Source: CAD feature listing. Evaluate the final solid. Frame: model axes, mm. A direction names the side the tool comes from. Give positions to 0.01 mm unless a question says otherwise; leave off trailing zeros. Write each loop counter-clockwise with the first axis right and the second up, starting at its lowest first coordinate (ties: lowest second). Pieces come first, ordered by that corner, then holes. Notation, with made-up numbers: (-26.75, 72.5) -> (-20.75, 72.5) arc R5 cw to (-20.75, 76.5) -> close; hole circle Ø7 at (-4.5, 49). An arc over 180 degrees is marked (long way). Use one line per item in the form item = value. Start each with the question number.
(1) Set-up query: faces 1 (the face through (35, 0, 23)), 2 (the face through (23.65, -49.45, -25.8)), 3 (the face through (15.02, 271.03, 47.69)), 4 (the face through (35, 0, -25)). Return all of +Z, -Z, +X, -X, +Y, -Y with unobstructed straight access to the full face (end or side cutting, diameter ignored); none if empty.
(2) Cut plane B-B, the plane z = -8. Output: boundary loops of the cut face in (x, y).
(3) Cut plane C-C, the plane y = 370. Output: boundary loops of the cut face in (x, z), and give its area (3 significant figures).
(4) Material intervals for line 1 along X through (y, z) = (0, -1); line 2 along X through (y, z) = (1.5, 18.5); line 3 along Y through (x, z) = (0, -15), sorted ascending. Write a range as from..to.
(5) Cut plane D-D, the plane y = -26.5. Output: boundary loops of the cut face in (x, z), and give its area (3 significant figures).
(6) First-contact query: P1, Ø2, axis at x = 7.5, y = 228.5, coming from the +Z side; P2, Ø6, axis at y = 285, z = -0.5, coming from the +X side; P3, Ø8, axis at x = -29, y = 278, coming from the +Z side. Flat tips, straight axial feed; report the tip coordinate or a pass-through.
(7) Cut plane A-A, the plane x = 15. Output: boundary loops of the cut face in (y, z), and give its area (3 significant figures).
from build123d import *

# Parameters (mm, degrees)
BOSS_EXTRUDE1_DEPTH      = 132
BOSS_EXTRUDE1_DEPTH_BACK = 80
SKETCH1_R                = 35
BOSS_EXTRUDE2_DEPTH      = 35
BOSS_EXTRUDE2_DEPTH_BACK = 35
SKETCH2_R                = 35
SKETCH3_R                = 52.5
BOSS_EXTRUDE3_DEPTH      = 20
SKETCH4_R                = 50
BOSS_EXTRUDE4_DEPTH      = 282
CUT_EXTRUDE1_DEPTH       = 427.390079622
CUT_EXTRUDE1_DEPTH_BACK  = 427.390079622
SKETCH5_R                = 20


with BuildPart() as part:
    # Sketch1 → Boss-Extrude1 (new, two sides: drawn at the far end of the back side and taken through both)
    with BuildSketch(Plane(origin=(0, 0, 0), x_dir=(1, 0, 0), z_dir=(0, 1, 0)).offset(-BOSS_EXTRUDE1_DEPTH_BACK)):
        with Locations(Location((0, 0, 0), (0, 0, 270))):
            Circle(SKETCH1_R)
    extrude(amount=BOSS_EXTRUDE1_DEPTH + BOSS_EXTRUDE1_DEPTH_BACK)

    # Sketch2 → Boss-Extrude2 (add, two sides: drawn at the far end of the back side and taken through both)
    with BuildSketch(Plane.XY.offset(-BOSS_EXTRUDE2_DEPTH_BACK)):
        Circle(SKETCH2_R)
    extrude(amount=BOSS_EXTRUDE2_DEPTH + BOSS_EXTRUDE2_DEPTH_BACK)

    # Sketch3 → Boss-Extrude3 (add)
    with BuildSketch(Plane(origin=(0, 132, 0), x_dir=(1, 0, 0), z_dir=(0, 1, 0))):
        with Locations(Location((0, 0, 0), (0, 0, 270))):
            Circle(SKETCH3_R)
    extrude(amount=-BOSS_EXTRUDE3_DEPTH)

    # Sketch4 → Boss-Extrude4 (add)
    with BuildSketch(Plane(origin=(0, 132, 0), x_dir=(1, 0, 0), z_dir=(0, 1, 0))):
        with Locations(Location((0, 0, 0), (0, 0, 270))):
            Circle(SKETCH4_R)
    extrude(amount=BOSS_EXTRUDE4_DEPTH)

    # Sketch5 → Cut-Extrude1 (cut, two sides: drawn at the far end of the back side and taken through both)
    with BuildSketch(Plane.XY.offset(35).offset(-CUT_EXTRUDE1_DEPTH_BACK)):
        Circle(SKETCH5_R)
    extrude(amount=CUT_EXTRUDE1_DEPTH + CUT_EXTRUDE1_DEPTH_BACK, mode=Mode.SUBTRACT)


solid = part.part
Geometry says:
q1.face_1 = +Z, +X
q1.face_2 = -Y
q1.face_3 = +Y
q1.face_4 = -Z, +X
q2.outline = (-51.89, 112) -> (-34.07, 112) -> (-34.07, 8) arc R35 ccw to (-34.07, -8) -> (-34.07, -80) -> (34.07, -80) -> (34.07, -8) arc R35 ccw to (34.07, 8) -> (34.07, 112) -> (51.89, 112) -> (51.89, 132) -> (49.36, 132) -> (49.36, 414) -> (-49.36, 414) -> (-49.36, 132) -> (-51.89, 132) -> close; hole circle Ø40 at (0, 0)
q3.outline = circle Ø100 at (0, 0)
q3.area = 7,850 mm^2
q4.line_1 = -35..-20, 20..35
q4.line_2 = -34.97..-19.94, 19.94..34.97
q4.line_3 = -80..-20, 20..414
q5.outline = (-22.86, -35) -> (22.86, -35) -> (22.86, -26.5) arc R35 ccw to (22.86, 26.5) -> (22.86, 35) -> (-22.86, 35) -> (-22.86, 26.5) arc R35 ccw to (-22.86, -26.5) -> close
q5.area = 4,090 mm^2
q6.P1 = 49.58
q6.P2 = 50
q6.P3 = 43.3
q7.outline = (-80, -31.62) -> (-31.62, -31.62) -> (-31.62, -35) -> (-13.23, -35) -> (-13.23, 35) -> (-31.62, 35) -> (-31.62, 31.62) -> (-80, 31.62) -> close; (13.23, -35) -> (31.62, -35) -> (31.62, -31.62) -> (112, -31.62) -> (112, -50.31) -> (132, -50.31) -> (132, -47.7) -> (414, -47.7) -> (414, 47.7) -> (132, 47.7) -> (132, 50.31) -> (112, 50.31) -> (112, 31.62) -> (31.62, 31.62) -> (31.62, 35) -> (13.23, 35) -> close
q7.area = 39,600 mm^2
